Model file for the job. Use its own axes, mm. Give positions to 0.01 mm unless a question says otherwise; leave off trailing zeros. Loops run counter-clockwise (first coordinate to the right, second up) from the corner with the lowest first, then second, coordinate; pieces in that order, holes last. Notation, with made-up numbers: (29.5, -23) - (44.5, -23) arc R33 ccw to (44.5, 16) - close; hole circle Ø6 at (20, 11). An arc over 180 degrees is marked (long way). Answer as CSV lines item,"result". Start each with the question number.
Item 1: Pin check, flat tip, straight feed: pin 1 (4 mm diameter, centred on x = 12.7, z = -38.1, fed in from -Y). Stop position of the tip, or through.
Item 2: Saw through at C-C on z = -88.9. Give the cut face in (x, y) (3 decimals), plus the area to 3 significant figures.
Item 3: Saw through at A-A on x = 12.7. Give the cut face in (y, z) (3 decimals).
Item 4: Saw through at D-D on y = 2.55. State how many separate pieces and enclosed holes the cut face has, plus the area to 3 significant figures.
Item 5: Drill centre lines: L1, parallel to X at y = 1.75, z = -12.7; L2, parallel to X at y = 1.65, z = -38.1; L3, parallel to X at y = 1.8, z = -88.9. Where is each one in solid material? Low to high. Write a range as from..to.
Item 6: Saw through at B-B on z = -114.3. Give the cut face in (x, y) (3 decimals), plus the area to 3 significant figures.
from build123d import *

# Parameters (mm, degrees)
SKETCH1_R           = 2.54
SKETCH1_R_2         = 14.2875
BOSS_EXTRUDE1_DEPTH = 3.175


with BuildPart() as part:
    # Sketch1 → Boss-Extrude1 (new body)
    with BuildSketch(Plane(origin=(0, 0, 0), x_dir=(1, 0, 0), z_dir=(0, 1, 0))):
        with BuildLine():
            Line((0, 6.35), (0, 120.65))
            ThreePointArc((0, 120.65), (1.859871939, 125.140128061), (6.35, 127))
            Line((6.35, 127), (23.4773747, 127))
            ThreePointArc((23.4773747, 127), (25.317504045, 126.727534368), (26.999720946, 125.933519369))
            Line((26.999720946, 125.933519369), (98.772346246, 78.085102503))
            ThreePointArc((98.772346246, 78.085102503), (100.848633702, 75.797880961), (101.6, 72.801583134))
            Line((101.6, 72.801583134), (101.6, 6.35))
            ThreePointArc((101.6, 6.35), (99.740128061, 1.859871939), (95.25, 0))
            Line((95.25, 0), (6.35, 0))
            ThreePointArc((6.35, 0), (1.859871939, 1.859871939), (0, 6.35))
        make_face()
        with Locations(Location((88.9, 12.7, 0), (0, 0, 270))):
            Circle(SKETCH1_R, mode=Mode.SUBTRACT)
        with Locations(Location((63.5, 12.7, 0), (0, 0, 270))):
            Circle(SKETCH1_R, mode=Mode.SUBTRACT)
        with Locations(Location((38.1, 12.7, 0), (0, 0, 270))):
            Circle(SKETCH1_R, mode=Mode.SUBTRACT)
        with Locations(Location((12.7, 12.7, 0), (0, 0, 270))):
            Circle(SKETCH1_R, mode=Mode.SUBTRACT)
        with Locations(Location((12.7, 38.1, 0), (0, 0, 270))):
            Circle(SKETCH1_R, mode=Mode.SUBTRACT)
        with Locations(Location((12.7, 63.5, 0), (0, 0, 270))):
            Circle(SKETCH1_R, mode=Mode.SUBTRACT)
        with Locations(Location((12.7, 88.9, 0), (0, 0, 270))):
            Circle(SKETCH1_R, mode=Mode.SUBTRACT)
        with Locations(Location((12.7, 114.3, 0), (0, 0, 270))):
            Circle(SKETCH1_R, mode=Mode.SUBTRACT)
        with Locations(Location((57.15, 76.2, 0), (0, 0, 270))):
            Circle(SKETCH1_R_2, mode=Mode.SUBTRACT)
    extrude(amount=BOSS_EXTRUDE1_DEPTH)


solid = part.part
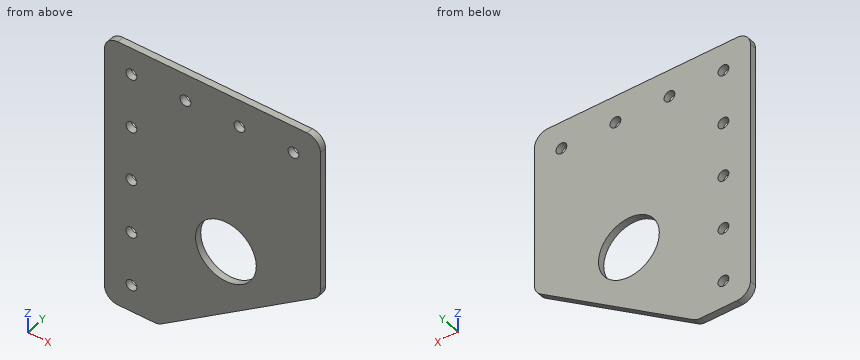
Responses:
1,pin 1,"through"
2,outline,"(0, 0) - (10.16, 0) - (10.16, 3.175) - (0, 3.175) - close; (15.24, 0) - (50.605, 0) - (50.605, 3.175) - (15.24, 3.175) - close; (63.695, 0) - (82.55, 0) - (82.55, 3.175) - (63.695, 3.175) - close"
2,area,"204 mm2"
3,outline,"(0, -127) - (3.175, -127) - (3.175, -116.84) - (0, -116.84) - close; (0, -111.76) - (3.175, -111.76) - (3.175, -91.44) - (0, -91.44) - close; (0, -86.36) - (3.175, -86.36) - (3.175, -66.04) - (0, -66.04) - close; (0, -60.96) - (3.175, -60.96) - (3.175, -40.64) - (0, -40.64) - close; (0, -35.56) - (3.175, -35.56) - (3.175, -15.24) - (0, -15.24) - close; (0, -10.16) - (3.175, -10.16) - (3.175, 0) - (0, 0) - close"
4,separate pieces,"1"
4,enclosed holes,"9"
4,area,"10,100 mm2"
5,L1,"0..10.16, 15.24..35.56, 40.64..60.96, 66.04..86.36, 91.44..101.6"
5,L2,"0..10.16, 15.24..101.6"
5,L3,"0..10.16, 15.24..50.6, 63.7..82.55"
6,outline,"(0, 0) - (10.16, 0) - (10.16, 3.175) - (0, 3.175) - close; (15.24, 0) - (44.45, 0) - (44.45, 3.175) - (15.24, 3.175) - close"
6,area,"125 mm2"
